Autodesk Inventor part; units mm, degrees
ref_plane "YZ Plane" through (0, 0, 0) normal (1, 0, 0) x (0, 1, 0)
ref_plane "XZ Plane" through (0, 0, 0) normal (0, 1, 0) x (-1, 0, 0)
ref_plane "XY Plane" through (0, 0, 0) normal (0, 0, 1) x (1, 0, 0)
sketch "Sketch1" plane through (0, 0, 0) normal (0, 0, 1) x (1, 0, 0)
  circle A0 centre (0, 0) radius 14.2875 construction
  line L0 (-35.56, 0) -> (35.56, 0)
  line L1 (0, -24.4475) -> (0, 24.4475)
  line L2 (-25.4, 17.4625) -> (25.4, 17.4625)
  line L3 (25.4, 17.4625) -> (25.4, -17.4625)
  line L4 (25.4, -17.4625) -> (-25.4, -17.4625)
  line L5 (-25.4, -17.4625) -> (-25.4, 17.4625)
  circle A1 centre (0, 0) radius 7.9375
  point P0 (0, 17.4625)
  point P1 (-25.4, 0)
  dimension "d0" = 28.575
  dimension "d1" = 50.8
  dimension "d2" = 34.925
  dimension "d3" = 15.875
extrude "Extrusion1" add sketch "Sketch1" along normal mid plane 6.35 contours L5 L2 L1 A1 L0 | L0 A1 L1 L4 L5 | L1 L2 L3 L0 A1 | A1 L0 L3 L4 L1
sketch "Sketch2" plane through (0, 0, -3.175) normal (0, 0, -1) x (-1, 0, 0)
  circle A0 centre (0, 0) radius 7.9375
  circle A1 centre (0, 0) radius 14.3256
  dimension "d6" = 28.6512
extrude "Bearing seat" cut sketch "Sketch2" against normal blind 2.54
sketch "Sketch3" plane through (0, 0, 3.175) normal (0, 0, 1) x (1, 0, 0)
  line L0 (-25.4, 17.4625) -> (25.4, 17.4625)
  line L1 (-25.4, -17.4625) -> (-25.4, 17.4625)
  line L2 (-35.56, 0) -> (35.56, 0)
  line L3 (0, -24.4475) -> (0, 24.4475)
  point P0 (-19.05, 11.1125)
  point P1 (19.05, 11.1125)
  point P2 (-19.05, -11.1125)
  point P3 (19.05, -11.1125)
  dimension "d9" = 6.35
  dimension "d10" = 6.35
hole "Hole1" at (-19.05, 11.1125, 3.175) at (19.05, 11.1125, 3.175) at (-19.05, -11.1125, 3.175) at (19.05, -11.1125, 3.175) direction (0, 0, -1) diameter 5.1054 end through all
properties part number "mount pillow block inner bearing capture"
Can you work these out from the model? Positions are in its coordinate system, mm. A direction names the side the tool comes from. Give positions to 0.01 mm unless a question says otherwise; leave off trailing zeros. Loops run counter-clockwise (first coordinate to the right, second up) from the corner with the lowest first, then second, coordinate; pieces in that order, holes last. Notation, with made-up numbers: (83, 23) - (140, 23) arc R32 cw to (140, 60) - close; hole circle Ø5 at (-4, 78). An arc over 180 degrees is marked (long way). Return JSON: item names as keys, results as strings.
1. For faces 1 (the face through (-6, -6, -0.635)), 2 (the face through (25.4, 0, 0)), which set-ups out of +Z, -Z, +X, -X, +Y, -Y let a thin tool reach every point of the face, with its end or its side?
Output values:
{"face 1": "-Z", "face 2": "+Z, -Z, +X, +Y, -Y"}
2. We'd pull the mould along Y, two halves only. Please class faces 3 (the face through (0, 17.462, 0)), 4 (the face through (-1.72, 7.75, 1.24)), 5 (the face through (5, 8, 3.175)), 6 (the face through (0, -17.462, 0)): +Y half, -Y half, draft (parallel to the pull), parting line (faces both ways), or undercut.
Output values:
{"face 3": "+Y half", "face 4": "undercut", "face 5": "draft", "face 6": "-Y half"}
3. If I drill on line 1 (Y direction, x = 19, z = -0.75); line 2 (X direction, y = -11.5, z = -2); line 3 (Y direction, x = 0, z = 1.5), over which ranges is the centre line in solid material (lowest first)?
Output values:
{"line 1": "y = -17.46 to -13.66, -8.56 to 8.56, 13.66 to 17.46", "line 2": "x = -25.4 to -21.57, -16.53 to -8.54, 8.54 to 16.53, 21.57 to 25.4", "line 3": "y = -17.46 to -7.94, 7.94 to 17.46"}
4. I want a section at D-D on x = 0. Please give me the cut outline in (y, z) (1 decimal), and give its area (3 significant figures).
Output values:
{"outline": "(-17.5, -3.2) - (-14.3, -3.2) - (-14.3, -0.6) - (-7.9, -0.6) - (-7.9, 3.2) - (-17.5, 3.2) - close; (7.9, -0.6) - (14.3, -0.6) - (14.3, -3.2) - (17.5, -3.2) - (17.5, 3.2) - (7.9, 3.2) - close", "area": "88.5 mm²"}
5. I'm going to push flat-ended pins straight in: pin 1 Ø4 at (x, y) = (19.05, 11.11) entering from -Z; pin 2 Ø14.5 at (x, y) = (0.5, -5) entering from -Z (3 decimals). Where does each tip first touch, or does it pass through?
Output values:
{"pin 1": "passes through", "pin 2": "stops at z = -0.635"}
6. I want a section at A-A on y = 0. Please give me the cut outline in (x, z) (1 decimal).
Output values:
{"outline": "(-25.4, -3.2) - (-14.3, -3.2) - (-14.3, -0.6) - (-7.9, -0.6) - (-7.9, 3.2) - (-25.4, 3.2) - close; (7.9, -0.6) - (14.3, -0.6) - (14.3, -3.2) - (25.4, -3.2) - (25.4, 3.2) - (7.9, 3.2) - close"}
7. I want a section at C-C on z = 2. Give the number of separate pieces and of enclosed holes in the cut face, and give its area (3 significant figures).
Output values:
{"separate pieces": "1", "enclosed holes": "5", "area": "1,490 mm²"}
8. I want a section at B-B on x = -19.05. Please give me the cut outline in (y, z) (1 decimal), and give its area (3 significant figures).
Output values:
{"outline": "(-17.5, -3.2) - (-13.7, -3.2) - (-13.7, 3.2) - (-17.5, 3.2) - close; (-8.6, -3.2) - (8.6, -3.2) - (8.6, 3.2) - (-8.6, 3.2) - close; (13.7, -3.2) - (17.5, -3.2) - (17.5, 3.2) - (13.7, 3.2) - close", "area": "157 mm²"}
